Geometry: final body of the model. Coordinates: model frame, mm. Face numbers are marked on the shaded views. A direction names the side the tool comes from. Round coordinates to 2 decimals unless told otherwise and drop trailing zeros. Loops run counter-clockwise (first coordinate to the right, second up) from the corner with the lowest first, then second, coordinate; pieces in that order, holes last. Notation, with made-up numbers: (15.5, 0.25) - (29.5, 0.25) arc R15 ccw to (29.5, 20.25) - close; hole circle Ø4 at (-27, 33). An arc over 180 degrees is marked (long way). Return JSON: item names as keys, results as strings. Group by question number.
1. Section D-D on z = -0.25. Return loops of the section in (x, y) (3 decimals).
2. Draft query along Y for the marked faces 1, 2 and 3. Return one class per face: +Y half, -Y half, draft (parallel to the pull), parting line (faces both ways), or undercut.
3. Section A-A on z = 2.5. Return loops of the section in (x, y) (3 decimals), and give its area (3 significant figures).
4. Material intervals for probe 1 along Y at (x, z) = (-2.25, 8); probe 2 along X at (y, z) = (-2, 4) (3 decimals); probe 3 along X at (y, z) = (-1.5, 7.5) (1 decimal), sorted ascending.
5. Set-up query: the marked faces 4, 5 and 6. Return all of +Z, -Z, +X, -X, +Y, -Y with unobstructed straight access to the full face (end or side cutting, diameter ignored); none if empty.
6. Section B-B on y = -0.75. Return loops of the section in (x, z) (3 decimals).
7. First-contact query: pin 1 Ø1 at (x, z) = (-2, 2) entering from -Y; pin 2 Ø0.5 at (y, z) = (-4, 6.5) entering from -X (3 decimals); pin 3 Ø1.2 at (x, y) = (3, 1) entering from -Z. Flat tips, straight axial feed; report the tip coordinate or a pass-through.
8. Section C-C on x = -1.5. Return loops of the section in (y, z).
from build123d import *

# Parameters (mm, degrees)
F0_W      = 6.95
F0_H      = 7
F1_DEPTH  = 8.23
F3_DEPTH  = 7.001
F4_W      = 2.9
F4_H      = 4.05
F5_DEPTH  = 1.1
F6_W      = 0.87
F6_H      = 0.57
F7_DEPTH  = 3
F8_W      = 0.87
F8_H      = 0.57
F9_DEPTH  = 3
F10_R     = 0.75
F11_DEPTH = 0.85
F12_W     = 1
F12_H     = 2.52
F13_DEPTH = 6.25
F14_R     = 0.875
F15_DEPTH = 1.5


with BuildPart() as f1:
    # F0 (on Top) → F1 (new body)
    with BuildSketch(Plane.XY):
        Rectangle(F0_W, F0_H)
    extrude(amount=F1_DEPTH)

    # F2 (on face) → F3 (cut, through all)
    with BuildSketch(Plane.XZ.offset(3.5)):
        Polygon((3.475, 8.23), (2.475, 8.23), (3.475, 5.37), align=None)
    extrude(amount=-F3_DEPTH, mode=Mode.SUBTRACT)

    # F4 (on face) → F5 (cut)
    with BuildSketch(Plane.YZ.offset(3.475)):
        with Locations((-1.7, 2.4635673035)):
            Rectangle(F4_W, F4_H)
        with Locations((1.7, 2.4635673035)):
            Rectangle(F4_W, F4_H)
    extrude(amount=-F5_DEPTH, mode=Mode.SUBTRACT)

    # F6 (on face) → F7 (join)
    with BuildSketch(Plane.XY.offset(8.23)):
        with Locations((1.47, -3.785)):
            Rectangle(F6_W, F6_H)
    extrude(amount=-F7_DEPTH)

    # F8 (on face) → F9 (cut)
    with BuildSketch(Plane.XY.offset(8.23)):
        with Locations((1.47, 3.215)):
            Rectangle(F8_W, F8_H)
    extrude(amount=-F9_DEPTH, mode=Mode.SUBTRACT)

    # F10 (on face) → F11 (cut)
    with BuildSketch(Plane.XY.offset(8.23)):
        with Locations((-0.595, -2.08)):
            Circle(F10_R)
        with Locations((-0.595, 2.08)):
            Circle(F10_R)
    extrude(amount=-F11_DEPTH, mode=Mode.SUBTRACT)

    # F12 (on face) → F13 (cut)
    with BuildSketch(Plane.XY.offset(8.23)):
        with Locations((-2.465, -1.62)):
            Rectangle(F12_W, F12_H)
        with Locations((-2.465, 1.62)):
            Rectangle(F12_W, F12_H)
    extrude(amount=-F13_DEPTH, mode=Mode.SUBTRACT)

    # F14 (on face) → F15 (join)
    with BuildSketch(Plane(origin=(0, 0, 0), x_dir=(1, 0, 0), z_dir=(0, 0, -1))):
        with Locations((0.225, 2.3)):
            Circle(F14_R)
        with Locations((0.225, -2.3)):
            Circle(F14_R)
    extrude(amount=F15_DEPTH)


solid = f1.part
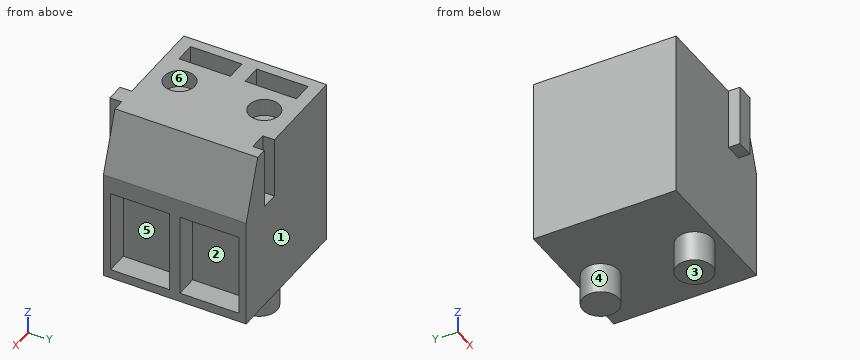
Taken from the geometry:
{
 "1": {"outline": "circle Ø1.75 at (0.225, -2.3); circle Ø1.75 at (0.225, 2.3)"},
 "2": {"face 1": "+Y half", "face 2": "undercut", "face 3": "draft"},
 "3": {"outline": "(-3.475, -3.5) - (3.475, -3.5) - (3.475, -3.15) - (2.375, -3.15) - (2.375, -0.25) - (3.475, -0.25) - (3.475, 0.25) - (2.375, 0.25) - (2.375, 3.15) - (3.475, 3.15) - (3.475, 3.5) - (-3.475, 3.5) - close; hole (-2.965, -2.88) - (-1.965, -2.88) - (-1.965, -0.36) - (-2.965, -0.36) - close; hole (-2.965, 0.36) - (-1.965, 0.36) - (-1.965, 2.88) - (-2.965, 2.88) - close", "area": "37.2 mm2"},
 "4": {"probe 1": "-3.5 to -2.88, -0.36 to 0.36, 2.88 to 3.5", "probe 2": "-3.475 to -2.965, -1.965 to 2.375", "probe 3": "-3.5 to -3, -2 to -1.1, -0.1 to 2.7"},
 "5": {"face 4": "-Z", "face 5": "+X", "face 6": "+Z"},
 "6": {"outline": "(-3.475, 0) - (3.475, 0) - (3.475, 0.439) - (2.375, 0.439) - (2.375, 4.489) - (3.475, 4.489) - (3.475, 5.37) - (2.475, 8.23) - (-1.965, 8.23) - (-1.965, 1.98) - (-2.965, 1.98) - (-2.965, 8.23) - (-3.475, 8.23) - close"},
 "7": {"pin 1": "y = -3.5", "pin 2": "x = 1.035", "pin 3": "z = 0"},
 "8": {"outline": "(-3.5, 0) - (3.5, 0) - (3.5, 8.23) - (-3.5, 8.23) - close"}
}
